Geometry check sheet. Reference: the model listing, model coordinates, mm. Give positions to 0.01 mm unless a question says otherwise; leave off trailing zeros. Write each loop counter-clockwise with the first axis right and the second up, starting at its lowest first coordinate (ties: lowest second). Pieces come first, ordered by that corner, then holes. Notation, with made-up numbers: (68, 54) - (124, 54) arc R14 cw to (124, 64) - close; hole circle Ø3 at (-19.75, -32). An arc over 180 degrees is marked (long way). Use a Markdown table: item, result.
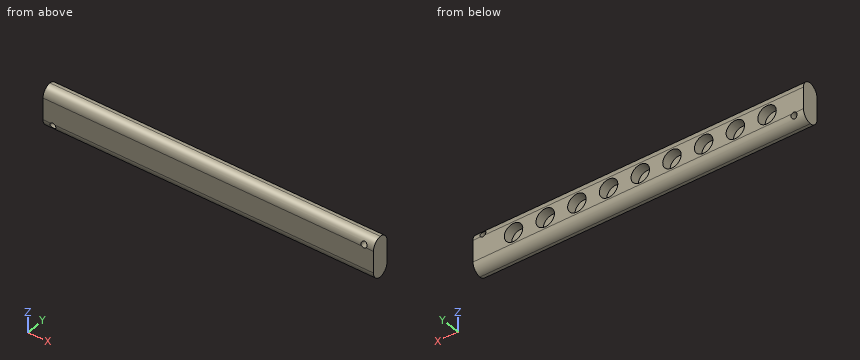
```python
from build123d import *

# Parameters (mm, degrees)
SKETCH1_W           = 340
SKETCH1_H           = 42.5
BOSS_EXTRUDE1_DEPTH = 41.5
SKETCH2_R           = 9.5
CUT_EXTRUDE1_DEPTH  = 10
SKETCH4_R           = 3.05
CUT_EXTRUDE3_DEPTH  = 301.787476707
CUT_EXTRUDE4_DEPTH  = 344.473796902
CUT_EXTRUDE5_DEPTH  = 344.473797021
CUT_EXTRUDE6_DEPTH  = 344.473797021


with BuildPart() as part:
    # Sketch1 → Boss-Extrude1 (new body)
    with BuildSketch(Plane(origin=(0, 0, 0), x_dir=(1, 0, 0), z_dir=(0, 1, 0))):
        with Locations((126.814516129, -4.284274194)):
            Rectangle(SKETCH1_W, SKETCH1_H)
    extrude(amount=BOSS_EXTRUDE1_DEPTH)

    # Sketch2 → Cut-Extrude1 (cut)
    with BuildSketch(Plane(origin=(0, 41.5, 0), x_dir=(1, 0, 0), z_dir=(0, 1, 0))):
        with Locations(Location((-5.685483871, -4.284274194, 0), (0, 0, 270))):
            Circle(SKETCH2_R)
        with Locations(Location((26.914516129, -4.284274194, 0), (0, 0, 270))):
            Circle(SKETCH2_R)
        with Locations(Location((59.514516129, -4.284274194, 0), (0, 0, 270))):
            Circle(SKETCH2_R)
        with Locations(Location((92.114516129, -4.284274194, 0), (0, 0, 270))):
            Circle(SKETCH2_R)
        with Locations(Location((124.714516129, -4.284274194, 0), (0, 0, 270))):
            Circle(SKETCH2_R)
        with Locations(Location((157.314516129, -4.284274194, 0), (0, 0, 270))):
            Circle(SKETCH2_R)
        with Locations(Location((189.914516129, -4.284274194, 0), (0, 0, 270))):
            Circle(SKETCH2_R)
        with Locations(Location((222.514516129, -4.284274194, 0), (0, 0, 270))):
            Circle(SKETCH2_R)
        with Locations(Location((255.114516129, -4.284274194, 0), (0, 0, 270))):
            Circle(SKETCH2_R)
    extrude(amount=-CUT_EXTRUDE1_DEPTH, mode=Mode.SUBTRACT)

    # Sketch4 → Cut-Extrude3 (cut, through all)
    with BuildSketch(Plane(origin=(0, 41.5, 0), x_dir=(1, 0, 0), z_dir=(0, 1, 0))):
        with Locations(Location((286.814516129, -17.534274194, 0), (0, 0, 270))):
            Circle(SKETCH4_R)
        with Locations(Location((-33.185483871, 8.965725806, 0), (0, 0, 270))):
            Circle(SKETCH4_R)
    extrude(amount=-CUT_EXTRUDE3_DEPTH, mode=Mode.SUBTRACT)

    # Sketch3 → Cut-Extrude4 (cut, through all)
    with BuildSketch(Plane.ZY.offset(43.185483871)):
        with BuildLine():
            Line((-6.965725806, 41.5), (-16.965725806, 41.5))
            Line((-16.965725806, 41.5), (-16.965725806, 31.5))
            ThreePointArc((-16.965725806, 31.5), (-14.036793618, 38.571067812), (-6.965725806, 41.5))
        make_face()
        with BuildLine():
            ThreePointArc((-6.965725806, 0), (-14.036793618, 2.928932188), (-16.965725806, 10))
            Line((-16.965725806, 10), (-16.965725806, 0))
            Line((-16.965725806, 0), (-6.965725806, 0))
        make_face()
        with BuildLine():
            Line((25.534274194, 0), (25.534274194, 10))
            ThreePointArc((25.534274194, 10), (22.605342005, 2.928932188), (15.534274194, 0))
            Line((15.534274194, 0), (25.534274194, 0))
        make_face()
        with BuildLine():
            Line((25.534274194, 41.5), (15.534274194, 41.5))
            ThreePointArc((15.534274194, 41.5), (22.605342005, 38.571067812), (25.534274194, 31.5))
            Line((25.534274194, 31.5), (25.534274194, 41.5))
        make_face()
    extrude(amount=-CUT_EXTRUDE4_DEPTH, mode=Mode.SUBTRACT)

    # Sketch5 → Cut-Extrude5 (cut, through all)
    with BuildSketch(Plane.ZY.offset(43.185483871)):
        with BuildLine():
            Line((25.534274194, 23.1), (4.284274194, 23.1))
            Line((4.284274194, 23.1), (-16.965725806, 23.1))
            Line((-16.965725806, 23.1), (-16.965725806, 10))
            ThreePointArc((-16.965725806, 10), (-14.036793618, 2.928932188), (-6.965725806, 0))
            Line((-6.965725806, 0), (15.534274194, 0))
            ThreePointArc((15.534274194, 0), (22.605342005, 2.928932188), (25.534274194, 10))
            Line((25.534274194, 10), (25.534274194, 23.1))
        make_face()
    extrude(amount=-CUT_EXTRUDE5_DEPTH, mode=Mode.SUBTRACT)

    # Sketch6 → Cut-Extrude6 (cut, through all)
    with BuildSketch(Plane.ZY.offset(43.185483871)):
        with BuildLine():
            ThreePointArc((-16.933674442, 32.3), (-16.957709752, 31.900320899), (-16.965725806, 31.5))
            Line((-16.965725806, 31.5), (-16.965725806, 23.1))
            Line((-16.965725806, 23.1), (-6.965725806, 23.1))
            ThreePointArc((-6.965725806, 23.1), (-13.74805579, 25.751530772), (-16.933674442, 32.3))
        make_face()
        with BuildLine():
            ThreePointArc((25.502222829, 32.3), (22.316604177, 25.751530772), (15.534274194, 23.1))
            Line((15.534274194, 23.1), (25.534274194, 23.1))
            Line((25.534274194, 23.1), (25.534274194, 31.5))
            ThreePointArc((25.534274194, 31.5), (25.52625814, 31.900320899), (25.502222829, 32.3))
        make_face()
    extrude(amount=-CUT_EXTRUDE6_DEPTH, mode=Mode.SUBTRACT)


solid = part.part
```
1) Depth check by flat-ended pin: P1, Ø1, axis at x = 259, z = 20.5, coming from the -Y side; P2, Ø2, axis at x = 219, y = 29.5, coming from the +Z side; P3, Ø1, axis at x = 168.5, y = 33, coming from the -Z side; P4, Ø21, axis at x = 60, z = 2, coming from the +Y side. Enter the tip coordinate at first touch or a pass-through.
Working result:
| item | result |
|---|---|
| P1 | stops at y = 24.15 |
| P2 | stops at z = 25.19 |
| P3 | stops at z = -16.92 |
| P4 | stops at y = 41.5 |
2) Material ranges on L1, parallel to Y at x = 63, z = 16.5; L2, parallel to Z at x = -28.5, y = 32.5; L3, parallel to Z at x = 161, y = 35, recorded low to high. Write a range as from..to.
Working result:
| item | result |
|---|---|
| L1 | y = 23.15..41.45 |
| L2 | z = -16.92..25.48 |
| L3 | z = -16.33..-4.47, 13.04..24.9 |
3) Section check A-A on x = 272.5. Record the boundary of the cut face in (y, z), then the cut area to 3 significant figures.
Working result:
| item | result |
|---|---|
| outline | (23.1, -6.97) arc R10 ccw to (32.3, -16.93) arc R10 ccw to (41.5, -6.97) - (41.5, 15.53) arc R10 ccw to (32.3, 25.5) arc R10 ccw to (23.1, 15.53) - close |
| area | 696 mm² |
